Check sheet for the modelled part. Datum: model origin and axes. Units: mm. A direction names the side the tool comes from. Round coordinates to 2 decimals unless told otherwise and drop trailing zeros. Write each loop counter-clockwise with the first axis right and the second up, starting at its lowest first coordinate (ties: lowest second). Pieces come first, ordered by that corner, then holes. Notation, with made-up numbers: M 43,55 L 84,55 A12 cw 84,70 Z; hole C 35,-1 d2. An arc over 180 degrees is marked long. Answer in a Markdown table with one row per item.
```python
from build123d import *

# Parameters (mm, degrees)
EXTRUDE_1_DEPTH     = 160
SKETCH_2_R          = 2.2
CUT_EXTRUDE_1_DEPTH = 16
SKETCH_3_R          = 2.2
CUT_EXTRUDE_2_DEPTH = 160


with BuildPart() as part:
    # ｽｹｯﾁ1 → ﾎﾞｽ - 押し出し1 (new body)
    with BuildSketch(Plane.XY):
        Polygon((0, 0), (0, 15), (1.5, 15), (1.5, 1.5), (15, 1.5), (15, 0), align=None)
    extrude(amount=EXTRUDE_1_DEPTH)

    # ｽｹｯﾁ2 → ｶｯﾄ - 押し出し1 (cut, through all)
    with BuildSketch(Plane.ZY):
        with Locations((20, 7.5)):
            Circle(SKETCH_2_R)
        with Locations((140, 7.5)):
            Circle(SKETCH_2_R)
    extrude(amount=-CUT_EXTRUDE_1_DEPTH, mode=Mode.SUBTRACT)

    # ｽｹｯﾁ3 → ｶｯﾄ - 押し出し2 (cut)
    with BuildSketch(Plane(origin=(0, 0, 0), x_dir=(-1, 0, 0), z_dir=(0, -1, 0))):
        with Locations((-7.5, -10)):
            Circle(SKETCH_3_R)
        with Locations((-7.5, -150)):
            Circle(SKETCH_3_R)
    extrude(amount=-CUT_EXTRUDE_2_DEPTH, mode=Mode.SUBTRACT)


solid = part.part
```
1. Scan lines: L1, parallel to Z at x = 7.5, y = 1.2; L2, parallel to X at y = 1, z = 10; L3, parallel to X at y = 5.5, z = 94. Record each from-to range of solid material in increasing order.
Found:
| item | result |
|---|---|
| L1 | z = 0 to 7.8, 12.2 to 147.8, 152.2 to 160 |
| L2 | x = 0 to 5.3, 9.7 to 15 |
| L3 | x = 0 to 1.5 |
2. Section check B-B, the plane x = 7.5. Record the cut outline in (y, z).
Found:
| item | result |
|---|---|
| outline | M 0,0 L 1.5,0 L 1.5,7.8 L 0,7.8 Z; M 0,12.2 L 1.5,12.2 L 1.5,147.8 L 0,147.8 Z; M 0,152.2 L 1.5,152.2 L 1.5,160 L 0,160 Z |
3. Go/stop test with flat-tipped pins: pin 1 (1.5 mm diameter, centred on x = 5, y = 4, fed in from +Z); pin 2 (4 mm diameter, centred on x = 11.5, z = 71, fed in from +Y). Record where each tip stops, or that it passes through.
Found:
| item | result |
|---|---|
| pin 1 | passes through |
| pin 2 | stops at y = 1.5 |
4. Draft check along Z on faces 1 (the face through (1.5, 8, 79)), 2 (the face through (6.317, 0.74, 148.145)), 3 (the face through (4, 1, 160)), 4 (the face through (4, 1, 0)). Enter one of: +Z half, -Z half, draft (parallel to the pull), parting line (faces both ways), or undercut.
Found:
| item | result |
|---|---|
| face 1 | draft |
| face 2 | undercut |
| face 3 | +Z half |
| face 4 | -Z half |
5. Section check A-A, the plane z = 150. Record the cut outline in (x, y), and give its area (4 significant figures).
Found:
| item | result |
|---|---|
| outline | M 0,0 L 5.3,0 L 5.3,1.5 L 1.5,1.5 L 1.5,15 L 0,15 Z; M 9.7,0 L 15,0 L 15,1.5 L 9.7,1.5 Z |
| area | 36.15 mm2 |
6. Section check D-D, the plane z = 106.5. Record the cut outline in (x, y), and give its area (4 significant figures).
Found:
| item | result |
|---|---|
| outline | M 0,0 L 15,0 L 15,1.5 L 1.5,1.5 L 1.5,15 L 0,15 Z |
| area | 42.75 mm2 |
7. Section check C-C, the plane y = 7.5. Record the cut outline in (x, z), and give its area (3 significant figures).
Found:
| item | result |
|---|---|
| outline | M 0,0 L 1.5,0 L 1.5,17.8 L 0,17.8 Z; M 0,22.2 L 1.5,22.2 L 1.5,137.8 L 0,137.8 Z; M 0,142.2 L 1.5,142.2 L 1.5,160 L 0,160 Z |
| area | 227 mm2 |
8. Access from +Z, -Z, +X, -X, +Y, -Y to the whole of each face (thin tool, end or side, straight path). Record for faces 5 (the face through (8, 0, 79)), 6 (the face through (8, 1.5, 79)).
Found:
| item | result |
|---|---|
| face 5 | +Z, -Z, +X, -X, -Y |
| face 6 | +Z, -Z, +X, +Y |
